Geometry: see drawing. Coordinates: mm, zero at the bounding-box minimum. Coordinates: 2 decimals unless noted, no trailing zeros. Order: outer loops, then holes, each group sorted by start corner. A loop starts at its lowest first (then second) coordinate and runs counter-clockwise, first axis right, second up. Notation, with made-up numbers: (9.5, 50.5) -> (38.5, 50.5) arc R20 ccw to (38.5, 87.5) -> close; hole circle Ø5 at (36, -23). An arc over 180 degrees is marked (long way). Use one line per item in the form item = value.
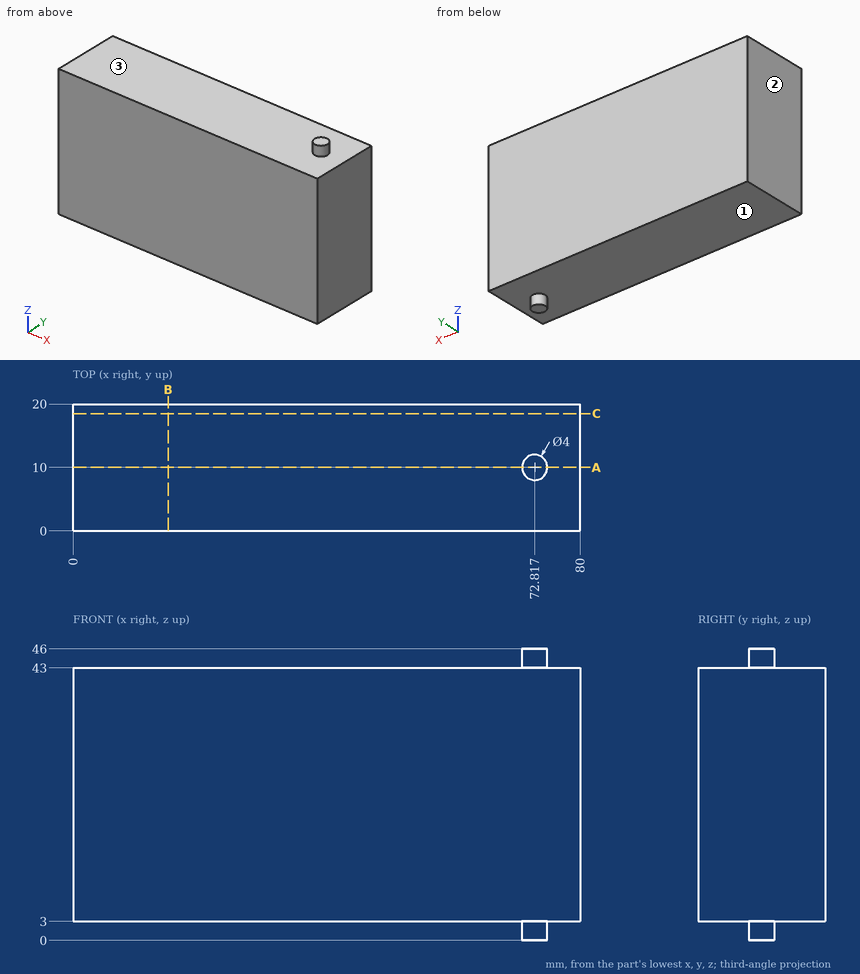
1) Pull-direction query (Z, two-part tool) for the marked faces 1, 2 and 3; classes: released by +Z, released by -Z, zero draft, split by the parting line, or undercut.
Results found:
face_1 = released by -Z
face_2 = zero draft
face_3 = released by +Z
2) Material intervals for probe 1 along Z at (x, y) = (4.5, 12.5), sorted ascending. Write a range as from..to.
Results found:
probe_1 = 3..43
3) Contact query for a flat-ended pin moving along its axis: P1, Ø8, axis at x = 44, y = 15.5, coming from the -Z side. Output: stop coordinate, or through.
Results found:
P1 = 3
4) Section B-B, the plane x = 15. Output: boundary loops of the cut face in (y, z).
Results found:
outline = (0, 3) -> (20, 3) -> (20, 43) -> (0, 43) -> close
5) Section A-A, the plane y = 10. Output: boundary loops of the cut face in (x, z).
Results found:
outline = (0, 3) -> (70.82, 3) -> (70.82, 0) -> (74.82, 0) -> (74.82, 3) -> (80, 3) -> (80, 43) -> (74.82, 43) -> (74.82, 46) -> (70.82, 46) -> (70.82, 43) -> (0, 43) -> close
6) Section C-C, the plane y = 18.5. Output: boundary loops of the cut face in (x, z), and give its area (3 significant figures).
Results found:
outline = (0, 3) -> (80, 3) -> (80, 43) -> (0, 43) -> close
area = 3,200 mm2
